Design review of the part built by this model. Coordinates are the model's own, in mm. Face numbers are marked on the shaded views. A direction names the side the tool comes from. Coordinates: 2 decimals unless noted, no trailing zeros. Loops run counter-clockwise (first coordinate to the right, second up) from the corner with the lowest first, then second, coordinate; pieces in that order, holes last. Notation, with made-up numbers: (6.25, 88.5) - (60.25, 88.5) arc R16 ccw to (60.25, 105.5) - close; hole circle Ø1 at (51, 39.5). An arc over 180 degrees is marked (long way). Return JSON: item names as keys, results as strings. Group by question number.
from build123d import *

# Parameters (mm, degrees)
SKETCH1_W           = 20
SKETCH1_H           = 30
BOSS_EXTRUDE1_DEPTH = 5
FILLET2_R           = 10
SKETCH2_R           = 2.5
CUT_EXTRUDE1_DEPTH  = 19.708286934
SKETCH3_W           = 6.666666667
SKETCH3_H           = 5
BOSS_EXTRUDE2_DEPTH = 5


with BuildPart() as part:
    # Sketch1 → Boss-Extrude1 (new body)
    with BuildSketch(Plane.XY):
        Rectangle(SKETCH1_W, SKETCH1_H)
    extrude(amount=BOSS_EXTRUDE1_DEPTH)

    # Fillet2
    fillet2_edges = [part.edges().sort_by_distance(p)[0] for p in [
        (-10, 15, 2.5),
        (10, 15, 2.5),
    ]]
    fillet(fillet2_edges, radius=FILLET2_R - 0.0001)  # a hair under: the kernel refuses the full size

    # Sketch2 → Cut-Extrude1 (cut, through all)
    with BuildSketch(Plane(origin=(0, 0, 0), x_dir=(-1, 0, 0), z_dir=(0, 0, -1))):
        with Locations((0, 5)):
            Circle(SKETCH2_R)
    extrude(amount=-CUT_EXTRUDE1_DEPTH, mode=Mode.SUBTRACT)

    # Sketch3 → Boss-Extrude2 (add)
    with BuildSketch(Plane.XZ.offset(15)):
        with Locations((-6.666666667, 2.5)):
            Rectangle(SKETCH3_W, SKETCH3_H)
        with Locations((6.666666667, 2.5)):
            Rectangle(SKETCH3_W, SKETCH3_H)
    extrude(amount=BOSS_EXTRUDE2_DEPTH)


solid = part.part
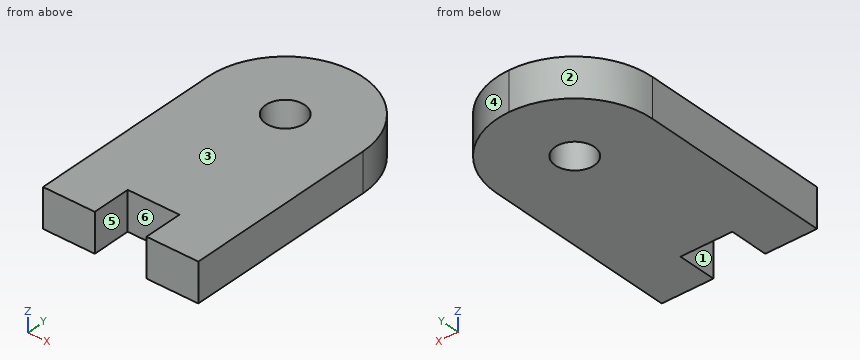
Item 1: Add section B-B (x = -1.5). State the section outline as (y, z) points, then the cut area to 3 significant figures.
Item 2: Add section D-D (x = 6.5). State the section outline as (y, z) points, then the cut area to 3 significant figures.
Item 3: For P1, Ø4.5, axis at x = 0, y = 5, coming from the +Z side; P2, Ø3, axis at x = 1, z = 1.5, coming from the -Y side, all flat-tipped, find the tip position at first contact; note any pin that passes through.
Item 4: To check wall thickness, follow line 1 (Y direction, x = 0, z = 1.95); line 2 (X direction, y = -18.5, z = 2.8); line 3 (Y direction, x = -0.75, z = 3.6). State the ranges of each line that lie inside material, in increasing order. Write a range as from..to.
Item 5: For the marked faces 1 and 2, list the 3-axis set-ups (+Z, -Z, +X, -X, +Y, -Y) from which the entire face can be reached by the end or side of a thin tool; tool diameter is ignored.
Item 6: Add section C-C (y = 5.5). State the section outline as (x, z) points, then the cut area to 3 significant figures.
Item 7: Draft analysis for pull direction X (two halves, no side actions). For the marked faces 3, 4, 5 and 6, state which applies: pulls with the +X half, pulls with the -X half, needs draft (parallel to the pull), parting line crosses it, or undercut.
Answers below:
{
 "1": {"outline": "(-15, 0) - (3, 0) - (3, 5) - (-15, 5) - close; (7, 0) - (14.89, 0) - (14.89, 5) - (7, 5) - close", "area": "129 mm^2"},
 "2": {"outline": "(-20, 0) - (12.6, 0) - (12.6, 5) - (-20, 5) - close", "area": "163 mm^2"},
 "3": {"P1": "passes through", "P2": "stops at y = -15"},
 "4": {"line 1": "y = -15..2.5, 7.5..15", "line 2": "x = -10..-3.33, 3.33..10", "line 3": "y = -15..2.62, 7.38..14.97"},
 "5": {"face 1": "+Z, -Z, -Y", "face 2": "+Z, -Z, -X, +Y"},
 "6": {"outline": "(-9.99, 0) - (-2.45, 0) - (-2.45, 5) - (-9.99, 5) - close; (2.45, 0) - (9.99, 0) - (9.99, 5) - (2.45, 5) - close", "area": "75.4 mm^2"},
 "7": {"face 3": "needs draft", "face 4": "pulls with the +X half", "face 5": "undercut", "face 6": "undercut"}
}
